Model file for the job. Use its own axes, mm. A direction names the side the tool comes from. Coordinates: 2 decimals unless noted, no trailing zeros. Write each loop counter-clockwise with the first axis right and the second up, starting at its lowest first coordinate (ties: lowest second). Pieces come first, ordered by that corner, then holes. Notation, with made-up numbers: M -3,63 L 26,63 A17 cw 26,76 Z; hole C 74,42 d6. An arc over 180 degrees is marked long. Answer in a Markdown table with one row per item. Add a question column.
```python
from build123d import *

# Parameters (mm, degrees)
SKETCH1_R           = 15
BOSS_EXTRUDE1_DEPTH = 50.8
SKETCH2_R           = 127
BOSS_EXTRUDE2_DEPTH = 203.2
BOSS_EXTRUDE3_START = -4
SKETCH3_R           = 2
BOSS_EXTRUDE3_DEPTH = 5
BOSS_EXTRUDE4_START = -15
SKETCH3_2_R         = 2
BOSS_EXTRUDE4_DEPTH = 5


with BuildPart() as part:
    # Sketch1 → Boss-Extrude1 (new body)
    with BuildSketch(Plane(origin=(0, 0, 0), x_dir=(0, 0, -1), z_dir=(1, 0, 0))):
        with BuildLine():
            ThreePointArc((-387.415853794, -91.706685848), (-404.293314152, -123.415853794), (-372.584146206, -140.293314152))
            Line((-372.584146206, -140.293314152), (-15.614846066, -31.32373832))
            ThreePointArc((-15.614846066, -31.32373832), (0, -35), (15.614846066, -31.32373832))
            Line((15.614846066, -31.32373832), (372.584146206, -140.293314152))
            ThreePointArc((372.584146206, -140.293314152), (404.293314152, -123.415853794), (387.415853794, -91.706685848))
            Line((387.415853794, -91.706685848), (30.446553653, 17.262889985))
            ThreePointArc((30.446553653, 17.262889985), (0, 35), (-30.446553653, 17.262889985))
            Line((-30.446553653, 17.262889985), (-387.415853794, -91.706685848))
        make_face()
        Circle(SKETCH1_R, mode=Mode.SUBTRACT)
    extrude(amount=BOSS_EXTRUDE1_DEPTH)

    # Sketch2 → Boss-Extrude2 (add)
    with BuildSketch(Plane(origin=(50.8, 0, 0), x_dir=(0, 0, -1), z_dir=(1, 0, 0))):
        with Locations((-380, -116)):
            Circle(SKETCH2_R)
    boss_extrude2 = extrude(amount=BOSS_EXTRUDE2_DEPTH)

    # Sketch3 → Boss-Extrude3 (add)
    with BuildSketch(Plane.ZY.offset(BOSS_EXTRUDE3_START)):
        with BuildLine():
            Line((372.826777317, -80.979847323), (371.07500083, -86.718425469))
            Line((371.07500083, -86.718425469), (385.421446196, -91.097866686))
            Line((385.421446196, -91.097866686), (387.173222683, -85.35928854))
            ThreePointArc((387.173222683, -85.35928854), (382.189720608, -75.996345249), (372.826777317, -80.979847323))
        make_face()
        with Locations((380, -83.169567931)):
            Circle(SKETCH3_R, mode=Mode.SUBTRACT)
    boss_extrude3 = extrude(amount=-BOSS_EXTRUDE3_DEPTH)

    # Sketch3<2> → Boss-Extrude4 (add)
    with BuildSketch(Plane.ZY.offset(BOSS_EXTRUDE4_START)):
        with BuildLine():
            Line((372.826777317, -80.979847323), (371.07500083, -86.718425469))
            Line((371.07500083, -86.718425469), (385.421446196, -91.097866686))
            Line((385.421446196, -91.097866686), (387.173222683, -85.35928854))
            ThreePointArc((387.173222683, -85.35928854), (382.189720608, -75.996345249), (372.826777317, -80.979847323))
        make_face()
        with Locations((380, -83.169567931)):
            Circle(SKETCH3_2_R, mode=Mode.SUBTRACT)
    boss_extrude4 = extrude(amount=-BOSS_EXTRUDE4_DEPTH)

    # Mirror1: Boss-Extrude2, Boss-Extrude3, Boss-Extrude4 across plane
    add(boss_extrude2.mirror(Plane.XY))
    add(boss_extrude3.mirror(Plane.XY))
    add(boss_extrude4.mirror(Plane.XY))


solid = part.part
```
1) Slice it at C-C (y = -116). Give the cut face in (x, z), then the cut area to 3 significant figures.
2) Slice it at D-D (x = 235). Give the cut face in (y, z), then the cut area to 3 significant figures.
3) Drill centre lines: probe 1 along Y at (x, z) = (17, -380); probe 2 along Y at (x, z) = (13.5, 0); probe 3 along X at (y, z) = (-142, 267). Where is each one in solid material? Low to high.
4) Two-plate mould, pull along Z, no slides. Class faces 3 (the face through (25.044, 34.996, -0.517)), 4 (the face through (50.8, -34, 4)), 5 (the face through (254, -114, 382)): released by +Z, released by -Z, zero draft, split by the parting line, or undercut.
5) Flat gauge pins, fed straight in: pin 1 Ø10 at (x, y) = (180, -86.5) entering from +Z; pin 2 Ø2 at (x, z) = (37.5, -393) entering from +Y; pin 3 Ø3 at (y, z) = (-101.5, 237) entering from +X; pin 4 Ø6 at (x, y) = (72, -76) entering from +Z. Where does each tip first touch, or does it go through?
6) Slice it at B-B (y = 0). Give the cut face in (x, z).
7) Slice it at A-A (z = 0). Give the cut face in (x, y).
8) Which spindle directions (+Z, -Z, +X, -X, +Y, -Y) get a long thin tool onto all of the face, cutting with end or side? Do faces 1 (the face through (25.044, -85.046, -191.601)), 2 (the face through (0, -27, 2)). Say none if no direction does.
Ans:
| question | item | result |
|---|---|---|
| 1 | outline | M 0,-405.4 L 50.8,-405.4 L 50.8,-507 L 254,-507 L 254,-253 L 50.8,-253 L 50.8,-293 L 0,-293 Z; M 0,293 L 50.8,293 L 50.8,253 L 254,253 L 254,507 L 50.8,507 L 50.8,405.4 L 0,405.4 Z |
| 1 | area | 115,000 mm2 |
| 2 | outline | C -116,-380 d254; C -116,380 d254 |
| 2 | area | 101,000 mm2 |
| 3 | probe 1 | y = -141.4 to -85.17, -81.17 to -75.67 |
| 3 | probe 2 | y = -35 to -15, 15 to 35 |
| 3 | probe 3 | x = 50.8 to 254 |
| 4 | face 3 | split by the parting line |
| 4 | face 4 | undercut |
| 4 | face 5 | zero draft |
| 5 | pin 1 | stops at z = 504.61 |
| 5 | pin 2 | stops at y = -93.61 |
| 5 | pin 3 | passes through |
| 5 | pin 4 | stops at z = 501.49 |
| 6 | outline | M 0,-87 L 50.8,-87 L 50.8,-15 L 0,-15 Z; M 0,15 L 50.8,15 L 50.8,87 L 0,87 Z; M 50.8,-431.7 L 254,-431.7 L 254,-328.3 L 50.8,-328.3 Z; M 50.8,328.3 L 254,328.3 L 254,431.7 L 50.8,431.7 Z |
| 7 | outline | M 0,-35 L 50.8,-35 L 50.8,-15 L 0,-15 Z; M 0,15 L 50.8,15 L 50.8,35 L 0,35 Z |
| 8 | face 1 | -X, -Y |
| 8 | face 2 | +Z, -Z, -X, +Y, -Y |
